Model file for the job. Use its own axes, mm. A direction names the side the tool comes from. Give positions to 0.01 mm unless a question says otherwise; leave off trailing zeros. Order: outer loops, then holes, each group sorted by start corner. A loop starts at its lowest first (then second) coordinate and runs counter-clockwise, first axis right, second up. Notation, with made-up numbers: (50, -8) - (102, -8) arc R31 cw to (102, 25) - close; hole circle Ø10 at (-25, 41.25). An arc over 180 degrees is marked (long way). Return JSON: item names as keys, results as strings. Group by question number.
from build123d import *

# Parameters (mm, degrees)
F0_W     = 92
F0_H     = 60
F1_DEPTH = 20
F2_W     = 18
F2_H     = 56
F2_W_2   = 28
F2_W_3   = 38
F3_DEPTH = 18


with BuildPart() as f1:
    # F0 (on Top) → F1 (new body)
    with BuildSketch(Plane.XY):
        Rectangle(F0_W, F0_H)
    extrude(amount=F1_DEPTH)

    # F2 (on face) → F3 (cut)
    with BuildSketch(Plane.XY.offset(20)):
        with Locations((-35, 0)):
            Rectangle(F2_W, F2_H)
        with Locations((-10, 0)):
            Rectangle(F2_W_2, F2_H)
        with Locations((25, 0)):
            Rectangle(F2_W_3, F2_H)
    extrude(amount=-F3_DEPTH, mode=Mode.SUBTRACT)


solid = f1.part
(1) Slice it at B-B (y = 24). Give the cut face in (x, z), and give its area (3 significant figures).
(2) Drill centre lines: L1, parallel to X at y = 25.5, z = 18; L2, parallel to Y at x = 24, z = 14.25; L3, parallel to Z at x = -39, y = -14. Where is each one in solid material? Low to high.
(3) Pull direction X, two halves, no side cores. Call faces 3 (the face through (-46, 0, 10)), 4 (the face through (-10, -28, 11)), 5 (the face through (-1, 30, 10)): released by +X, released by -X, zero draft, split by the parting line, or undercut.
(4) Drop a flat-ended pin along its axis: pin 1 Ø5.5 at (x, y) = (-37.5, 3) entering from +Z. Give the stop position or say it passes through.
(5) 3-axis set-ups, long thin cutter, end or side, ignore diameter. For faces 1 (the face through (-10, 0, 2)), 2 (the face through (-1, 0, 0)): which of +Z, -Z, +X, -X, +Y, -Y reach the whole face in a straight line?
(6) Slice it at A-A (z = 5.75). Give the cut face in (x, y), and give its area (3 significant figures).
(7) Slice it at C-C (x = 24.5). Give the cut face in (y, z).
Result set:
{
 "1": {"outline": "(-46, 0) - (46, 0) - (46, 20) - (44, 20) - (44, 2) - (6, 2) - (6, 20) - (4, 20) - (4, 2) - (-24, 2) - (-24, 20) - (-26, 20) - (-26, 2) - (-44, 2) - (-44, 20) - (-46, 20) - close", "area": "328 mm²"},
 "2": {"L1": "x = -46 to -44, -26 to -24, 4 to 6, 44 to 46", "L2": "y = -30 to -28, 28 to 30", "L3": "z = 0 to 2"},
 "3": {"face 3": "released by -X", "face 4": "undercut", "face 5": "zero draft"},
 "4": {"pin 1": "stops at z = 2"},
 "5": {"face 1": "+Z", "face 2": "-Z, +X, -X, +Y, -Y"},
 "6": {"outline": "(-46, -30) - (46, -30) - (46, 30) - (-46, 30) - close; hole (-44, -28) - (-26, -28) - (-26, 28) - (-44, 28) - close; hole (-24, -28) - (4, -28) - (4, 28) - (-24, 28) - close; hole (6, -28) - (44, -28) - (44, 28) - (6, 28) - close", "area": "816 mm²"},
 "7": {"outline": "(-30, 0) - (30, 0) - (30, 20) - (28, 20) - (28, 2) - (-28, 2) - (-28, 20) - (-30, 20) - close"}
}
